Autodesk Inventor part; units mm, degrees
ref_plane "YZ Plane" through (0, 0, 0) normal (1, 0, 0) x (0, 1, 0)
ref_plane "XZ Plane" through (0, 0, 0) normal (0, 1, 0) x (-1, 0, 0)
ref_plane "XY Plane" through (0, 0, 0) normal (0, 0, 1) x (1, 0, 0)
sketch "Sketch1" plane through (0, 0, 0) normal (0, 1, 0) x (-1, 0, 0)
  line L0 (-30, 30) -> (30, 30)
  line L1 (30, 30) -> (30, -30)
  line L2 (30, -30) -> (-30, -30)
  line L3 (-30, -30) -> (-30, 30)
  line L4 (-30, 30) -> (30, -30) construction
  line L5 (30, 30) -> (-30, -30) construction
  point P0 (0, 0)
  dimension "d0" = 60
  dimension "d1" = 60
extrude "Extrusion1" add sketch "Sketch1" along normal blind 70
sketch "Sketch2" plane through (0, 70, 0) normal (0, 1, 0) x (1, 0, 0)
  line L0 (22.5, 22.5) -> (-22.5, 22.5)
  line L1 (-22.5, 22.5) -> (-22.5, -22.5)
  line L2 (-22.5, -22.5) -> (22.5, -22.5)
  line L3 (22.5, -22.5) -> (22.5, 22.5)
  line L4 (22.5, 22.5) -> (-22.5, -22.5) construction
  line L5 (-22.5, 22.5) -> (22.5, -22.5) construction
  point P0 (0, 0)
  dimension "d4" = 45
  dimension "d5" = 45
extrude "Extrusion2" cut sketch "Sketch2" against normal blind 60
sketch "Sketch3" plane through (-30, 0, 30) normal (0, 0, 1) x (1, 0, 0)
  circle A0 centre (30, 40) radius 21.5
  point P0 (30, 0)
  dimension "d8" = 43
extrude "Extrusion3" cut sketch "Sketch3" against normal blind 15
sketch "Sketch4" plane through (30, 0, 30) normal (1, 0, 0) x (0, 0, -1)
  circle A0 centre (30, 40) radius 21.5
  point P0 (30, 0)
  dimension "d11" = 43
extrude "Extrusion4" cut sketch "Sketch4" against normal blind 15
sketch "Sketch5" plane through (0, 0, 0) normal (0, -1, 0) x (1, 0, 0)
  point P0 (0, 0)
  point P1 (0, 0)
hole "Hole1" at (0, 0, 0) direction (0, 1, 0) diameter 3.302 depth 8
sketch "Sketch7" plane through (-30, 0, 30) normal (0, 0, 1) x (1, 0, 0)
  line L0 (11.5, 21.5) -> (48.5, 21.5)
  line L1 (48.5, 21.5) -> (48.5, 58.5)
  line L2 (48.5, 58.5) -> (11.5, 58.5)
  line L3 (11.5, 58.5) -> (11.5, 21.5)
  line L4 (11.5, 21.5) -> (48.5, 58.5) construction
  line L5 (48.5, 21.5) -> (11.5, 58.5) construction
  point P0 (30, 0)
  point P1 (30, 40)
  dimension "d21" = 37
  dimension "d22" = 37
hole "Hole2" at (-18.5, 58.5, 30) at (18.5, 58.5, 30) at (18.5, 21.5, 30) at (-18.5, 21.5, 30) direction (0, 0, -1) diameter 3.302 depth 6
sketch "Sketch8" plane through (30, 0, 30) normal (1, 0, 0) x (0, 0, -1)
  line L0 (11.5, 21.5) -> (48.5, 21.5)
  line L1 (48.5, 21.5) -> (48.5, 58.5)
  line L2 (48.5, 58.5) -> (11.5, 58.5)
  line L3 (11.5, 58.5) -> (11.5, 21.5)
  line L4 (11.5, 21.5) -> (48.5, 58.5) construction
  line L5 (48.5, 21.5) -> (11.5, 58.5) construction
  point P0 (30, 0)
  point P1 (30, 40)
  dimension "d30" = 37
  dimension "d31" = 37
hole "Hole3" at (30, 58.5, 18.5) at (30, 58.5, -18.5) at (30, 21.5, 18.5) at (30, 21.5, -18.5) direction (-1, 0, 0) diameter 3.302 depth 6
properties part number "immersion_chamber_bath"
Here's how the part is built. I have some questions about the finished solid (model axes, mm). A direction names the side the tool comes from. Round coordinates to 2 decimals unless told otherwise and drop trailing zeros. Loops run counter-clockwise (first coordinate to the right, second up) from the corner with the lowest first, then second, coordinate; pieces in that order, holes last. Notation, with made-up numbers: (65, 18.5) - (120, 18.5) arc R26 cw to (120, 34.5) - close; hole circle Ø2 at (27, 46.5). An arc over 180 degrees is marked (long way). One line per question, with ' | ' between items. Start each with the question number.
Q1. For faces 1 (the flat face through (0, 40, -22.5)), 2 (the cylindrical face through (27, 23.1, 18.9)), 3 (the cylindrical face through (0.632, 4.056, -1.525)), 4 (the cylindrical face through (-17.495, 59.81, 26.958)), which set-ups out of +Z, -Z, +X, -X, +Y, -Y let a thin tool reach every point of the face, with its end or its side?
Q2. Will these pins go through, and if not, where does the flat tip stop? pin 1 (12 mm diameter, centred on x = 2.5, z = 18.5, fed in from -Y); pin 2 (1.7 mm diameter, centred on x = -18.5, y = 58.5, fed in from +Z); pin 3 (6 mm diameter, centred on x = 5.5, y = 46.5, fed in from +Z); pin 4 (2.5 mm diameter, centred on y = 21.5, z = 18.5, fed in from +X).
Q3. I want a section at C-C (z = -12). Write out the boundary of the cut face in (x, y).
Q4. I want a section at A-A (x = 25). Write out the boundary of the cut face in (y, z), then the cut area to 3 significant figures.
Q5. I want a section at D-D (x = 0). Write out the boundary of the cut face in (y, z), then the cut area to 3 significant figures.
Q6. I want a section at B-B (y = 34.5). Write out the boundary of the cut face in (x, z), then the cut area to 3 significant figures.
Q7. We'd pull the mould along X, two halves only. Please class faces 5 (the flat face through (-30, 35, 0)), 6 (the cylindrical face through (26.958, 58.004, -20.075)), 7 (the flat face through (22.5, 60, 10)), 8 (the flat face through (24, 58, 19)): +X half, -X half, draft (parallel to the pull), parting line (faces both ways), or undercut.
Q8. Please list where these lines run through material, in increasing order: line 1 (Z direction, x = -22, y = 52); line 2 (X direction, y = 4.5, z = 0); line 3 (Z direction, x = 27.5, y = 58.5). Write a range as [from, to].
Response values:
1) face 1: +Y | face 2: +X | face 3: -Y | face 4: +Z
2) pin 1: stops at y = 0 | pin 2: stops at z = 24 | pin 3: stops at z = -22.5 | pin 4: stops at x = 24
3) outline: (-30, 0) - (30, 0) - (30, 22.16) - (22.5, 22.16) - (22.5, 10) - (-22.5, 10) - (-22.5, 70) - (-30, 70) - close; (22.5, 57.84) - (30, 57.84) - (30, 70) - (22.5, 70) - close
4) outline: (0, -30) - (70, -30) - (70, 30) - (0, 30) - close; hole circle Ø43 at (40, 0); hole circle Ø3.3 at (21.5, -18.5); hole circle Ø3.3 at (21.5, 18.5); hole circle Ø3.3 at (58.5, -18.5); hole circle Ø3.3 at (58.5, 18.5) | area: 2,710 mm²
5) outline: (0, -30) - (70, -30) - (70, -22.5) - (10, -22.5) - (10, 22.5) - (18.5, 22.5) - (18.5, 30) - (0, 30) - (0, 1.65) - (8, 1.65) - (8, -1.65) - (0, -1.65) - close; (61.5, 22.5) - (70, 22.5) - (70, 30) - (61.5, 30) - close | area: 1,150 mm²
6) outline: (-30, -30) - (30, -30) - (30, -20.78) - (22.5, -20.78) - (22.5, -22.5) - (-22.5, -22.5) - (-22.5, 22.5) - (-20.78, 22.5) - (-20.78, 30) - (-30, 30) - close; (20.78, 22.5) - (22.5, 22.5) - (22.5, 20.78) - (30, 20.78) - (30, 30) - (20.78, 30) - close | area: 951 mm²
7) face 5: -X half | face 6: draft | face 7: undercut | face 8: +X half
8) line 1: z = [-30, -22.5], [22.5, 30] | line 2: x = [-30, -1.65], [1.65, 30] | line 3: z = [-30, -20.15], [-16.85, -10.95], [10.95, 16.85], [20.15, 30]
